Source: CAD feature listing. Evaluate the final solid. Frame: model axes, mm. A direction names the side the tool comes from. Give positions to 0.01 mm unless a question says otherwise; leave off trailing zeros. Order: outer loops, then holes, each group sorted by start corner. A loop starts at its lowest first (then second) coordinate and runs counter-clockwise, first axis right, second up. Notation, with made-up numbers: M 77,2.5 L 121,2.5 A30 ccw 121,39.5 Z; hole C 67.25,83 d4. An arc over 180 degrees is marked long. Answer in a Markdown table with one row per item. Add a question column.
(1) Pin query (flat end, axial travel): P1, Ø1.5, axis at y = 5.5, z = -6.5, coming from the -X side. Return the tip coordinate at first contact, or that it passes through.
(2) Material intervals for line 1 along Z through (x, y) = (0, 5); line 2 along Z through (x, y) = (3, 7.5), sorted ascending.
(3) Mould query, pull axis X, two halves, no side actions, for faces 3 (the face through (-3, 0, 5)), 4 (the face through (-11.99, 7.69, -0.53)), 5 (the face through (-1.08, 4.44, 4.88)). Classes: pulls with the +X half, pulls with the -X half, needs draft (parallel to the pull), parting line crosses it, or undercut.
(4) Section query B-B, the plane x = 0. Return loops of the section in (y, z).
(5) Section query D-D, the plane y = 7.5. Return loops of the section in (x, z), plus the area to 3 significant figures.
(6) Section query C-C, the plane y = 3.5. Return loops of the section in (x, z).
(7) Set-up query: faces 1 (the face through (-11.19, 4.47, -0.49)), 2 (the face through (-11.99, 1.29, -0.53)). Return all of +Z, -Z, +X, -X, +Y, -Y with unobstructed straight access to the full face (end or side cutting, diameter ignored); none if empty.
(8) Section query A-A, the plane z = 0. Return loops of the section in (x, y).
from build123d import *

# Parameters (mm, degrees)
SKETCH_1_R      = 12
SKETCH_1_R_2    = 5
EXTRUDE_1_DEPTH = 9
CHAMFER_1_SIZE  = 0.6
FILLET_1_R      = 0.5
CHAMFER_2_SIZE  = 0.5


with BuildPart() as part:
    # 草图1 → 凸台-拉伸1 (new body)
    with BuildSketch(Plane(origin=(0, 0, 0), x_dir=(1, 0, 0), z_dir=(0, 1, 0))):
        Circle(SKETCH_1_R)
        Circle(SKETCH_1_R_2, mode=Mode.SUBTRACT)
    extrude(amount=EXTRUDE_1_DEPTH)

    # 倒角1
    chamfer_1_edges = [part.edges().sort_by_distance(p)[0] for p in [
        (-12, 0, 0),
        (-12, 9, 0),
    ]]
    chamfer(chamfer_1_edges, length=CHAMFER_1_SIZE)

    # 草图2 → 切除-旋转1 (revolve, cut)
    with BuildSketch(Plane.XY):
        Polygon((12, 6.5), (11.2, 6.5), (11.2, 2.5), (12, 2.5), (14.67598619, 3.734930545), align=None)
    revolve(axis=Axis((0, 0, 0), (0, 1, 0)), mode=Mode.SUBTRACT)

    # 圆角1
    fillet_1_edges = [part.edges().sort_by_distance(p)[0] for p in [
        (-12, 6.5, 0),
        (-12, 2.5, 0),
    ]]
    fillet(fillet_1_edges, radius=FILLET_1_R)

    # 倒角2
    chamfer_2_edges = [part.edges().sort_by_distance(p)[0] for p in [
        (-5, 0, 0),
        (-5, 9, 0),
    ]]
    chamfer(chamfer_2_edges, length=CHAMFER_2_SIZE)


solid = part.part
Values follow:
| question | item | result |
|---|---|---|
| 1 | P1 | stops at x = -9.61 |
| 2 | line 1 | z = -11.2 to -5, 5 to 11.2 |
| 2 | line 2 | z = -11.62 to -4, 4 to 11.62 |
| 3 | face 3 | needs draft |
| 3 | face 4 | parting line crosses it |
| 3 | face 5 | undercut |
| 4 | outline | M 0,-11.4 L 0.6,-12 L 2,-12 A0.5 ccw 2.5,-11.5 L 2.5,-11.2 L 6.5,-11.2 L 6.5,-11.5 A0.5 ccw 7,-12 L 8.4,-12 L 9,-11.4 L 9,-5.5 L 8.5,-5 L 0.5,-5 L 0,-5.5 Z; M 0,5.5 L 0.5,5 L 8.5,5 L 9,5.5 L 9,11.4 L 8.4,12 L 7,12 A0.5 ccw 6.5,11.5 L 6.5,11.2 L 2.5,11.2 L 2.5,11.5 A0.5 ccw 2,12 L 0.6,12 L 0,11.4 Z |
| 5 | outline | C 0,0 d24; hole C 0,0 d10 |
| 5 | area | 374 mm² |
| 6 | outline | C 0,0 d22.4; hole C 0,0 d10 |
| 7 | face 1 | none |
| 7 | face 2 | +Y, -Y |
| 8 | outline | M -12,0.6 L -11.4,0 L -5.5,0 L -5,0.5 L -5,8.5 L -5.5,9 L -11.4,9 L -12,8.4 L -12,7 A0.5 ccw -11.5,6.5 L -11.2,6.5 L -11.2,2.5 L -11.5,2.5 A0.5 ccw -12,2 Z; M 5,0.5 L 5.5,0 L 11.4,0 L 12,0.6 L 12,2 A0.5 ccw 11.5,2.5 L 11.2,2.5 L 11.2,6.5 L 11.5,6.5 A0.5 ccw 12,7 L 12,8.4 L 11.4,9 L 5.5,9 L 5,8.5 Z |
